from build123d import *

# Parameters (mm, degrees)
EXTRUIR_L_MINA1_START   = -30
EXTRUIR_L_MINA1_DEPTH   = 60
CROQUIS2_W              = 29.989677058
CROQUIS2_H              = 58.075247638
SALIENTE_EXTRUIR1_DEPTH = 30
CROQUIS3_R              = 7
CORTAR_EXTRUIR1_DEPTH   = 60
CROQUIS4_R              = 11
CORTAR_EXTRUIR2_DEPTH   = 7
CORTAR_EXTRUIR3_START   = -7
CROQUIS5_R              = 11
CORTAR_EXTRUIR3_DEPTH   = 7
CROQUIS7_R              = 2.65
CORTAR_EXTRUIR4_DEPTH   = 30
CROQUIS8_R              = 5
CORTAR_EXTRUIR5_DEPTH   = 3
CROQUIS9_R              = 5
CORTAR_EXTRUIR6_DEPTH   = 3
CROQUIS10_R             = 5
CORTAR_EXTRUIR7_DEPTH   = 3
CROQUIS11_R             = 5
CORTAR_EXTRUIR8_DEPTH   = 3


# Read off the part's stored shape, not the designer's step: Extruir-Lámina1
with BuildPart() as part:
    # Extruir-Lámina1 outline → Extruir-Lámina1 (new body)
    with BuildSketch(Plane(origin=(0, 0, 0), x_dir=(0, 0, -1), z_dir=(1, 0, 0)).offset(EXTRUIR_L_MINA1_START)):
        Polygon((10.020236328, -26.000123541), (0.000367551, -26.000123541), (0.000367551, -36.000123541), (10.000367551, -36.000123541), (10.000367551, -56.000123541), (14.000367551, -56.000123541), (21.74906786, -18.707636838), (22, -16.2665), (22, 16.2665), (21.74906786, 18.707636838), (14.000367551, 56.000123541), (10.000367551, 56.000123541), (10.000367551, 36.000123541), (-10.000367551, 36.000123541), (-10.000367551, 56.000123541), (-14.000367551, 56.000123541), (-21.74906786, 18.707636838), (-22, 16.2665), (-22, -16.2665), (-21.74906786, -18.707636838), (-14.000367551, -56.000123541), (-10.000367551, -56.000123541), (-10.000367551, -36.000123541), (-0.000367551, -36.000123541), (-0.000367551, -26.000123541), (-10.020236328, -26.000123541), (-11.853902107, -17.175165292), (-12, -15.753884831), (-12, 15.753884831), (-11.853902107, 17.175165292), (-10.020236328, 26.000123541), (10.020236328, 26.000123541), (11.853902107, 17.175165292), (12, 15.753884831), (12, -15.753884831), (11.853902107, -17.175165292), align=None)
    extrude(amount=EXTRUIR_L_MINA1_DEPTH)

    # Croquis2 → Saliente-Extruir1 (add, symmetric)
    with BuildSketch(Plane(origin=(0, 0, 0), x_dir=(0, 0, -1), z_dir=(1, 0, 0))):
        Rectangle(CROQUIS2_W, CROQUIS2_H)
    extrude(amount=SALIENTE_EXTRUIR1_DEPTH, both=True)

    # Croquis3 → Cortar-Extruir1 (cut)
    with BuildSketch(Plane.XY.offset(22)):
        Circle(CROQUIS3_R)
    extrude(amount=-CORTAR_EXTRUIR1_DEPTH, mode=Mode.SUBTRACT)

    # Croquis4 → Cortar-Extruir2 (cut)
    with BuildSketch(Plane.XY.offset(22)):
        Circle(CROQUIS4_R)
    extrude(amount=-CORTAR_EXTRUIR2_DEPTH, mode=Mode.SUBTRACT)

    # Croquis5 → Cortar-Extruir3 (cut)
    with BuildSketch(Plane(origin=(0, 0, -22), x_dir=(-1, 0, 0), z_dir=(0, 0, -1)).offset(CORTAR_EXTRUIR3_START)):
        with Locations(Location((0, 0, 0), (0, 0, 180))):
            Circle(CROQUIS5_R)
    extrude(amount=CORTAR_EXTRUIR3_DEPTH, mode=Mode.SUBTRACT)

    # Croquis7 → Cortar-Extruir4 (cut, symmetric)
    with BuildSketch(Plane.XY):
        with Locations(Location((-18, 46.000123541, 0), (0, 0, 270))):
            Circle(CROQUIS7_R)
        with Locations(Location((18, 46.000123541, 0), (0, 0, 270))):
            Circle(CROQUIS7_R)
        with Locations(Location((-18, -46.000123541, 0), (0, 0, 90))):
            Circle(CROQUIS7_R)
        with Locations(Location((18, -46.000123541, 0), (0, 0, 90))):
            Circle(CROQUIS7_R)
    extrude(amount=CORTAR_EXTRUIR4_DEPTH, both=True, mode=Mode.SUBTRACT)

    # Croquis8 → Cortar-Extruir5 (cut)
    with BuildSketch(Plane(origin=(0, 5.106275996, 24.575183206), x_dir=(1, 0, 0), z_dir=(0, 0.20343669587104055, 0.979088101640028))):
        with Locations(Location((-18, 41.767280673, 0), (0, 0, 270))):
            Circle(CROQUIS8_R)
        with Locations(Location((18, 41.767280673, 0), (0, 0, 270))):
            Circle(CROQUIS8_R)
    extrude(amount=-CORTAR_EXTRUIR5_DEPTH, mode=Mode.SUBTRACT)

    # Croquis9 → Cortar-Extruir6 (cut)
    with BuildSketch(Plane(origin=(0, -5.106275996, 24.575183206), x_dir=(1, 0, 0), z_dir=(0, -0.2034366958710477, 0.9790881016400266))):
        with Locations(Location((-18, -41.767280673, 0), (0, 0, 270))):
            Circle(CROQUIS9_R)
        with Locations(Location((18, -41.767280673, 0), (0, 0, 270))):
            Circle(CROQUIS9_R)
    extrude(amount=-CORTAR_EXTRUIR6_DEPTH, mode=Mode.SUBTRACT)

    # Croquis10 → Cortar-Extruir7 (cut)
    with BuildSketch(Plane(origin=(0, 5.106275996, -24.575183206), x_dir=(-1, 0, 0), z_dir=(0, 0.2034366958710399, -0.9790881016400281))):
        with Locations(Location((-18, 41.767280673, 0), (0, 0, 90))):
            Circle(CROQUIS10_R)
        with Locations(Location((18, 41.767280673, 0), (0, 0, 90))):
            Circle(CROQUIS10_R)
    extrude(amount=-CORTAR_EXTRUIR7_DEPTH, mode=Mode.SUBTRACT)

    # Croquis11 → Cortar-Extruir8 (cut)
    with BuildSketch(Plane(origin=(0, -5.106275996, -24.575183206), x_dir=(-1, 0, 0), z_dir=(0, -0.20343669587104735, -0.9790881016400267))):
        with Locations(Location((-18, -41.767280673, 0), (0, 0, 90))):
            Circle(CROQUIS11_R)
        with Locations(Location((18, -41.767280673, 0), (0, 0, 90))):
            Circle(CROQUIS11_R)
    extrude(amount=-CORTAR_EXTRUIR8_DEPTH, mode=Mode.SUBTRACT)


solid = part.part
Read the model definition and answer for the solid it produces. Units are mm, in the model's axes. A direction names the side the tool comes from. Round coordinates to 2 decimals unless told otherwise and drop trailing zeros. Order: outer loops, then holes, each group sorted by start corner. A loop starts at its lowest first (then second) coordinate and runs counter-clockwise, first axis right, second up.
1) For faces 1 (the face through (18.07, -43.146, 13.607)), 2 (the face through (0, -46, 10)), 3 (the face through (0, 46, 10)), determine the directions among +Z, -Z, +X, -X, +Y, -Y from which every point of the face is accessible in a straight line to the end or side of a thin tool.
2) The part is cut by section C-C on y = -22. Write down the section's boundary in (x, z), plus the area to 3 significant figures.
3) The part is cut by section D-D on y = 29. Write down the section's boundary in (x, z), plus the area to 3 significant figures.
4) The part is cut by section B-B on x = -18. Give the number of separate pieces and of enclosed holes in the cut face, plus the area to 3 significant figures.
5) The part is cut by section A-A on y = 0. Write down the section's boundary in (x, z).
6) Flat-ended cylindrical pins translate along their axes: pin 1 (22 mm diameter, centred on x = -1, y = -45, fed in from +Z); pin 2 (16 mm diameter, centred on x = -10, z = -1.5, fed in from +Y); pin 3 (2 mm diameter, centred on x = 11.5, y = -33, fed in from +Z); pin 4 (5 mm diameter, centred on x = -18, y = 46, fed in from -Z). Find the tip coordinate at first contact, or state that the pin passes through.
7) Straight lines are drawn through the part: L1, parallel to Y at x = 18, z = 11; L2, parallel to Y at x = -26, z = -4.5; L3, parallel to X at y = -3, z = 4.5. For each, find the intervals that lie inside material, in ascending order.
8) The mould has two halves that part along Y. Classify faces 4 (the face through (0, 46, -10)), 5 (the face through (-0.42, 17.47, -21.876)), 6 (the face through (-2.38, 10.74, -18.45)): released by +Y, released by -Y, zero draft, split by the parting line, or undercut.
Resolved:
1. face 1: none
1. face 2: +X, -X, -Y
1. face 3: +X, -X, +Y
2. outline: (-30, -21.06) - (30, -21.06) - (30, 21.06) - (-30, 21.06) - close
2. area: 2,530 mm2
3. outline: (-30, -19.61) - (30, -19.61) - (30, 19.61) - (-30, 19.61) - close
3. area: 2,350 mm2
4. separate pieces: 5
4. enclosed holes: 0
4. area: 3,330 mm2
5. outline: (-30, -22) - (-11, -22) - (-11, -15) - (-7, -15) - (-7, 15) - (-11, 15) - (-11, 22) - (-30, 22) - close; (7, -15) - (11, -15) - (11, -22) - (30, -22) - (30, 22) - (11, 22) - (11, 15) - (7, 15) - close
6. pin 1: stops at z = 18.57
6. pin 2: stops at y = 36
6. pin 3: stops at z = 18.99
6. pin 4: passes through
7. L1: y = -56 to -48.65, -43.35 to 43.35, 48.65 to 56
7. L2: y = -36 to 36
7. L3: x = -30 to -6.32, 6.32 to 30
8. face 4: zero draft
8. face 5: released by +Y
8. face 6: undercut
